Design review of the part shown in the three views and the two pictorial views. Dimensions are in mm from the part's minimum x, y and z. A direction names the side the tool comes from. Coordinates: 2 decimals unless noted, no trailing zeros. Write each loop counter-clockwise with the first axis right and the second up, starting at its lowest first coordinate (ties: lowest second). Pieces come first, ordered by that corner, then holes. Notation, with made-up numbers: (48, 86) - (100, 86) arc R17 cw to (100, 106) - close; hole circle Ø3 at (10.25, 37.25). An arc over 180 degrees is marked (long way). Write each question's results on one line, items separated by ' | '.
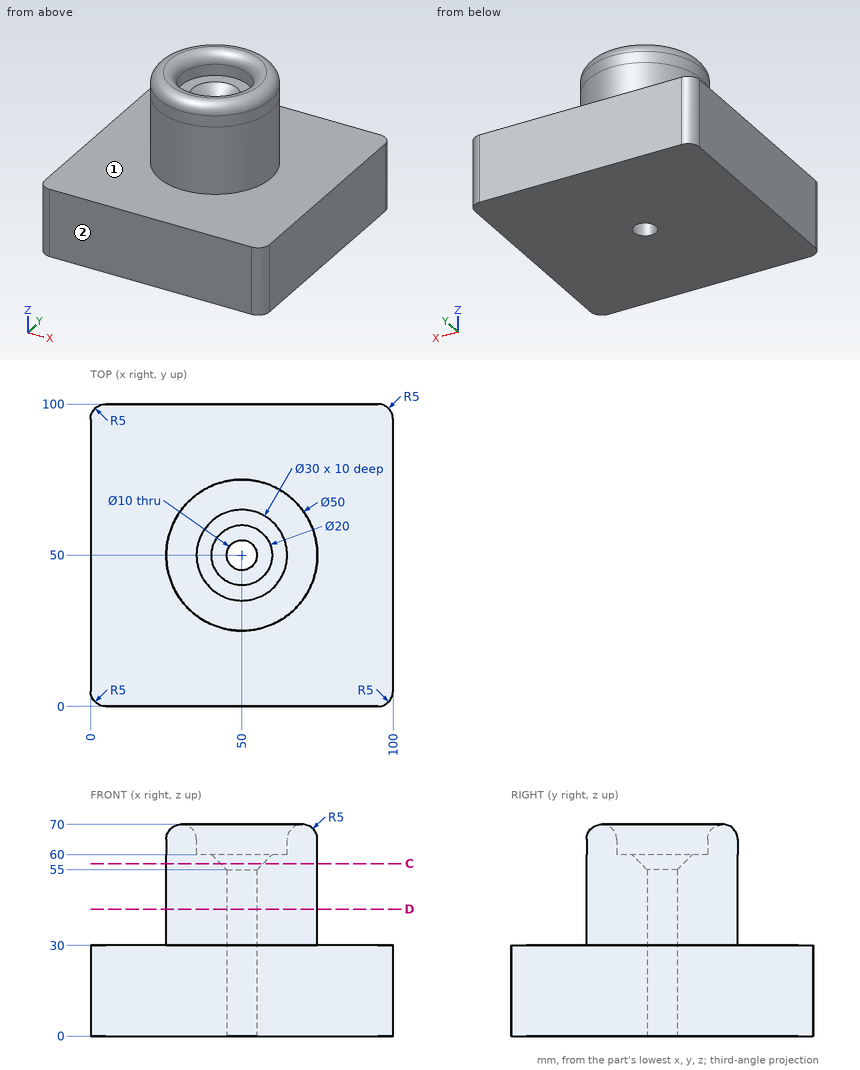
Q1. For the marked faces 1 and 2, list the 3-axis set-ups (+Z, -Z, +X, -X, +Y, -Y) from which the entire face can be reached by the end or side of a thin tool; tool diameter is ignored.
Results found:
face 1: +Z | face 2: +Z, -Z, +X, -X, -Y
Q2. Take a section at C-C on z = 57. State the section outline as (x, y) points, plus the area to 3 significant figures.
Results found:
outline: circle Ø50 at (50, 50); hole circle Ø14 at (50, 50) | area: 1,810 mm2
Q3. Wall thickness on line 1 along Y through (x, z) = (50, 32); line 2 along Y through (x, z) = (50, 26): over which ranges is each line inside the solid? List them lowest first. Write a range as from..to.
Results found:
line 1: 25..45, 55..75 | line 2: 0..45, 55..100
Q4. Take a section at D-D on z = 42. State the section outline as (x, y) points.
Results found:
outline: circle Ø50 at (50, 50); hole circle Ø10 at (50, 50)
Q5. For pin 1 (11.5 mm diameter, centred on x = 50, y = 50, fed in from +Z); pin 2 (24 mm diameter, centred on x = 50, y = 50, fed in from +Z); pin 3 (3 mm diameter, centred on y = 71, z = 52, fed in from +X), all flat-tipped, find the tip position at first contact; note any pin that passes through.
Results found:
pin 1: z = 55.75 | pin 2: z = 60 | pin 3: x = 65.64
